Build history of the part. All positions in model axes, mm. A direction names the side the tool comes from. Give positions to 0.01 mm unless a question says otherwise; leave off trailing zeros. Order: outer loops, then holes, each group sorted by start corner. A loop starts at its lowest first (then second) coordinate and runs counter-clockwise, first axis right, second up. Notation, with made-up numbers: (27, 52.25) - (58, 52.25) arc R19 ccw to (58, 65.25) - close; hole circle Ø5 at (87.5, 45.5). An arc over 180 degrees is marked (long way). Use a Markdown table: item, result. Add a question column.
(1) Slice it at A-A (z = 6). Write the cut outline in (x, y).
(2) Wall check: line 1 (X direction, y = -25, z = 34); line 2 (Z direction, x = 5.5, y = 66.5); line 3 (X direction, y = 1.5, z = 37). Give the ranges that are in metal, low to high.
(3) Slice it at B-B (x = 0). Write the cut outline in (y, z), then the cut area to 3 significant figures.
(4) Flat gauge pins, fed straight in: pin 1 (3 mm diameter, centred on x = -47, y = 42, fed in from +Z); pin 2 (1.5 mm diameter, centred on x = -23, y = 32.5, fed in from -Z); pin 3 (11 mm diameter, centred on y = 42.5, z = 5, fed in from -X). Where does each tip first touch, or does it go through?
(5) Which spindle directions (+Z, -Z, +X, -X, +Y, -Y) get a long thin tool onto all of the face, cutting with end or side? Do faces 1 (the face through (-8, 2, 22)), 2 (the face through (35.31, 17.17, 4.93)), 3 (the face through (18, -4, 45)). Say none if no direction does.
(6) Slice it at D-D (y = 35). Write the cut outline in (x, z), then the cut area to 3 significant figures.
(7) Mould opens along Y. For faces 4 (the face through (-0.99, -49.98, 22.18)), 5 (the face through (-1, 33, 25)), 6 (the face through (-34.81, 17.58, 4.93)), 7 (the face through (35.069, -67.425, 12.36)) say: +Y half, -Y half, draft (parallel to the pull), parting line (faces both ways), or undercut.
(8) Slice it at C-C (y = -5). Write the cut outline in (x, z).
from build123d import *

# Parameters (mm, degrees)
SKETCH1_R           = 73
BOSS_EXTRUDE1_DEPTH = 25
BOSS_EXTRUDE2_START = 2.5
SKETCH1_3_R         = 76
SKETCH1_3_R_2       = 73
BOSS_EXTRUDE2_DEPTH = 20
BOSS_EXTRUDE3_DEPTH = 45
CUT_EXTRUDE1_DEPTH  = 10


with BuildPart() as part:
    # Sketch1 → Boss-Extrude1 (new body)
    # profile 1 of 3: a face of its own
    with BuildSketch(Plane.XY):
        Circle(SKETCH1_R)
        with BuildLine():
            ThreePointArc((-12.5, 49.636176323), (-13.722739792, 52.053064023), (-16.394230769, 52.49980188))
            ThreePointArc((-16.394230769, 52.49980188), (-44.089289769, 32.880610208), (-54.995016416, 0.740384615))
            ThreePointArc((-54.995016416, 0.740384615), (-52.697492054, -2.21666073), (-49.305876787, -0.629310345))
            ThreePointArc((-49.305876787, -0.629310345), (-35.057623034, 17.378804457), (-14.698275862, 27.999629118))
            ThreePointArc((-14.698275862, 27.999629118), (-13.111991163, 29.074639736), (-12.5, 30.890517979))
            Line((-12.5, 30.890517979), (-12.5, 49.636176323))
        make_face(mode=Mode.SUBTRACT)
        with BuildLine():
            ThreePointArc((49.305876787, -0.629310345), (52.697492054, -2.21666073), (54.995016416, 0.740384615))
            ThreePointArc((54.995016416, 0.740384615), (44.089289769, 32.880610208), (16.394230769, 52.49980188))
            ThreePointArc((16.394230769, 52.49980188), (13.722739792, 52.053064023), (12.5, 49.636176323))
            Line((12.5, 49.636176323), (12.5, 30.890517979))
            ThreePointArc((12.5, 30.890517979), (13.111991163, 29.074639736), (14.698275862, 27.999629118))
            ThreePointArc((14.698275862, 27.999629118), (35.057623034, 17.378804457), (49.305876787, -0.629310345))
        make_face(mode=Mode.SUBTRACT)
        with BuildLine():
            ThreePointArc((-28.498326366, 3.06858376), (0, -65), (28.498326366, 3.06858376))
            ThreePointArc((28.498326366, 3.06858376), (23.895232771, 14.5315925), (12.5, 19.3))
            Line((12.5, 19.3), (-12.5, 19.3))
            ThreePointArc((-12.5, 19.3), (-23.895232771, 14.5315925), (-28.498326366, 3.06858376))
        make_face(mode=Mode.SUBTRACT)
    # profile 2 of 3: a face of its own
    with BuildSketch(Plane.XY):
        with BuildLine():
            Line((-12.5, 49.636176323), (-12.5, 30.890517979))
            ThreePointArc((-12.5, 30.890517979), (-13.111991163, 29.074639736), (-14.698275862, 27.999629118))
            ThreePointArc((-14.698275862, 27.999629118), (-35.057623034, 17.378804457), (-49.305876787, -0.629310345))
            ThreePointArc((-49.305876787, -0.629310345), (-52.697492054, -2.21666073), (-54.995016416, 0.740384615))
            ThreePointArc((-54.995016416, 0.740384615), (-44.089289769, 32.880610208), (-16.394230769, 52.49980188))
            ThreePointArc((-16.394230769, 52.49980188), (-13.722739792, 52.053064023), (-12.5, 49.636176323))
        make_face()
    # profile 3 of 3: a face of its own
    with BuildSketch(Plane.XY):
        with BuildLine():
            ThreePointArc((49.305876787, -0.629310345), (35.057623034, 17.378804457), (14.698275862, 27.999629118))
            ThreePointArc((14.698275862, 27.999629118), (13.111991163, 29.074639736), (12.5, 30.890517979))
            Line((12.5, 30.890517979), (12.5, 49.636176323))
            ThreePointArc((12.5, 49.636176323), (13.722739792, 52.053064023), (16.394230769, 52.49980188))
            ThreePointArc((16.394230769, 52.49980188), (44.089289769, 32.880610208), (54.995016416, 0.740384615))
            ThreePointArc((54.995016416, 0.740384615), (52.697492054, -2.21666073), (49.305876787, -0.629310345))
        make_face()
    extrude(amount=BOSS_EXTRUDE1_DEPTH)

    # Sketch1_3 → Boss-Extrude2 (add)
    with BuildSketch(Plane.XY.offset(BOSS_EXTRUDE2_START)):
        Circle(SKETCH1_3_R)
        Circle(SKETCH1_3_R_2, mode=Mode.SUBTRACT)
    extrude(amount=BOSS_EXTRUDE2_DEPTH)

    # Sketch1_4 → Boss-Extrude3 (add)
    with BuildSketch(Plane.XY):
        with BuildLine():
            ThreePointArc((-28.498326366, 3.06858376), (-23.895232771, 14.5315925), (-12.5, 19.3))
            Line((-12.5, 19.3), (12.5, 19.3))
            ThreePointArc((12.5, 19.3), (23.895232771, 14.5315925), (28.498326366, 3.06858376))
            ThreePointArc((28.498326366, 3.06858376), (0, -65), (-28.498326366, 3.06858376))
        make_face()
        with BuildLine():
            ThreePointArc((-8, -1.314561435), (0, -50), (8, -1.314561435))
            Line((8, -1.314561435), (8, 4.3))
            Line((8, 4.3), (-8, 4.3))
            Line((-8, 4.3), (-8, -1.314561435))
        make_face(mode=Mode.SUBTRACT)
    extrude(amount=BOSS_EXTRUDE3_DEPTH)

    # Sketch1_5 → Cut-Extrude1 (cut)
    with BuildSketch(Plane.XY):
        with BuildLine():
            ThreePointArc((49.305876787, -0.629310345), (35.057623034, 17.378804457), (14.698275862, 27.999629118))
            ThreePointArc((14.698275862, 27.999629118), (13.111991163, 29.074639736), (12.5, 30.890517979))
            Line((12.5, 30.890517979), (12.5, 49.636176323))
            ThreePointArc((12.5, 49.636176323), (13.722739792, 52.053064023), (16.394230769, 52.49980188))
            ThreePointArc((16.394230769, 52.49980188), (44.089289769, 32.880610208), (54.995016416, 0.740384615))
            ThreePointArc((54.995016416, 0.740384615), (52.697492054, -2.21666073), (49.305876787, -0.629310345))
        make_face()
        with BuildLine():
            Line((-12.5, 49.636176323), (-12.5, 30.890517979))
            ThreePointArc((-12.5, 30.890517979), (-13.111991163, 29.074639736), (-14.698275862, 27.999629118))
            ThreePointArc((-14.698275862, 27.999629118), (-35.057623034, 17.378804457), (-49.305876787, -0.629310345))
            ThreePointArc((-49.305876787, -0.629310345), (-52.697492054, -2.21666073), (-54.995016416, 0.740384615))
            ThreePointArc((-54.995016416, 0.740384615), (-44.089289769, 32.880610208), (-16.394230769, 52.49980188))
            ThreePointArc((-16.394230769, 52.49980188), (-13.722739792, 52.053064023), (-12.5, 49.636176323))
        make_face()
    extrude(amount=CUT_EXTRUDE1_DEPTH, mode=Mode.SUBTRACT)


solid = part.part
Solution:
| question | item | result |
|---|---|---|
| 1 | outline | circle Ø152 at (0, 0); hole (-55, 0.74) arc R3 ccw to (-49.31, -0.63) arc R55 cw to (-14.7, 28) arc R3 ccw to (-12.5, 30.89) - (-12.5, 49.64) arc R3 ccw to (-16.39, 52.5) arc R55 ccw to start; hole (-8, -1.31) arc R25 ccw (long way) to (8, -1.31) - (8, 4.3) - (-8, 4.3) - close; hole (12.5, 30.89) arc R3 ccw to (14.7, 28) arc R55 cw to (49.31, -0.63) arc R3 ccw to (55, 0.74) arc R55 ccw to (16.39, 52.5) arc R3 ccw to (12.5, 49.64) - close |
| 2 | line 1 | -40 to -25, 25 to 40 |
| 2 | line 2 | 0 to 25 |
| 2 | line 3 | -29.96 to -8, 8 to 29.96 |
| 3 | outline | (-76, 2.5) - (-73, 2.5) - (-73, 0) - (-50, 0) - (-50, 45) - (-65, 45) - (-65, 25) - (-73, 25) - (-73, 22.5) - (-76, 22.5) - close; (4.3, 0) - (73, 0) - (73, 2.5) - (76, 2.5) - (76, 22.5) - (73, 22.5) - (73, 25) - (19.3, 25) - (19.3, 45) - (4.3, 45) - close |
| 3 | area | 3,010 mm2 |
| 4 | pin 1 | z = 25 |
| 4 | pin 2 | z = 10 |
| 4 | pin 3 | x = -66.39 |
| 5 | face 1 | +Z, -Z |
| 5 | face 2 | -Z |
| 5 | face 3 | +Z, +X, -X, +Y, -Y |
| 6 | outline | (-67.46, 2.5) - (-64.06, 2.5) - (-64.06, 0) - (-42.43, 0) - (-42.43, 10) - (-12.5, 10) - (-12.5, 0) - (12.5, 0) - (12.5, 10) - (42.43, 10) - (42.43, 0) - (64.06, 0) - (64.06, 2.5) - (67.46, 2.5) - (67.46, 22.5) - (64.06, 22.5) - (64.06, 25) - (-64.06, 25) - (-64.06, 22.5) - (-67.46, 22.5) - close |
| 6 | area | 2,740 mm2 |
| 7 | face 4 | undercut |
| 7 | face 5 | draft |
| 7 | face 6 | undercut |
| 7 | face 7 | parting line |
| 8 | outline | (-75.84, 2.5) - (-72.83, 2.5) - (-72.83, 0) - (-15, 0) - (-15, 45) - (-34.64, 45) - (-34.64, 25) - (-72.83, 25) - (-72.83, 22.5) - (-75.84, 22.5) - close; (15, 0) - (72.83, 0) - (72.83, 2.5) - (75.84, 2.5) - (75.84, 22.5) - (72.83, 22.5) - (72.83, 25) - (34.64, 25) - (34.64, 45) - (15, 45) - close |
